Geometry check sheet. Reference: the model listing, model coordinates, mm. Coordinates: 2 decimals unless noted, no trailing zeros. Write each loop counter-clockwise with the first axis right and the second up, starting at its lowest first coordinate (ties: lowest second). Pieces come first, ordered by that corner, then holes.
from build123d import *

# Parameters (mm, degrees)
SKETCH1_W           = 15
SKETCH1_H           = 220
SKETCH1_W_2         = 519.948861259
SKETCH1_H_2         = 15
BOSS_EXTRUDE1_DEPTH = 20
BOSS_EXTRUDE3_DEPTH = 110
SKETCH3_R           = 7.5
CUT_EXTRUDE1_DEPTH  = 655.346046928
BOSS_EXTRUDE5_DEPTH = 10


with BuildPart() as part:
    # Sketch1 → Boss-Extrude1 (new body)
    with BuildSketch(Plane(origin=(0, 0, 0), x_dir=(1, 0, 0), z_dir=(0, 1, 0))):
        with Locations((72.505405333, -7.5)):
            Rectangle(SKETCH1_W, SKETCH1_H)
        with Locations((607.454266592, 0)):
            Rectangle(SKETCH1_W, SKETCH1_H)
        with Locations((339.979835963, 72.5)):
            Rectangle(SKETCH1_W_2, SKETCH1_H_2)
        with Locations((339.979835963, -87.5)):
            Rectangle(SKETCH1_W_2, SKETCH1_H_2)
    extrude(amount=-BOSS_EXTRUDE1_DEPTH)

    # Sketch2 → Boss-Extrude3 (add, symmetric)
    with BuildSketch(Plane.XY):
        with BuildLine():
            Line((145.005405333, 0), (185.005405333, 0))
            Line((185.005405333, 0), (185.005405333, -20))
            ThreePointArc((185.005405333, -20), (165.005392368, -39.99997407), (145.005405333, -19.99997407))
            Line((145.005405333, -19.99997407), (145.005405333, 0))
        make_face()
        with BuildLine():
            Line((494.954266592, 0), (534.954266592, 0))
            Line((534.954266592, 0), (534.954266592, -20))
            ThreePointArc((534.954266592, -20), (514.954261153, -39.999989122), (494.954266592, -19.999989122))
            Line((494.954266592, -19.999989122), (494.954266592, 0))
        make_face()
    extrude(amount=BOSS_EXTRUDE3_DEPTH, both=True)

    # Sketch3 → Cut-Extrude1 (cut, through all)
    with BuildSketch(Plane.XY.offset(110)):
        with Locations((165.005405333, -19.99997407)):
            Circle(SKETCH3_R)
        with Locations((514.954266592, -19.999989122)):
            Circle(SKETCH3_R)
    extrude(amount=-CUT_EXTRUDE1_DEPTH, mode=Mode.SUBTRACT)

    # Sketch4 → Boss-Extrude5 (add)
    with BuildSketch(Plane(origin=(0, 0, 0), x_dir=(1, 0, 0), z_dir=(0, 1, 0))):
        with BuildLine():
            Line((158.022043154, -30), (158.022043154, 30))
            ThreePointArc((158.022043154, 30), (163.022043154, 35), (168.022043154, 30))
            Line((168.022043154, 30), (168.022043154, -30))
            ThreePointArc((168.022043154, -30), (163.022043154, -35), (158.022043154, -30))
        make_face()
        with BuildLine():
            Line((508.880344162, -30), (508.880344162, 30))
            ThreePointArc((508.880344162, 30), (513.880344162, 35), (518.880344162, 30))
            Line((518.880344162, 30), (518.880344162, -30))
            ThreePointArc((518.880344162, -30), (513.880344162, -35), (508.880344162, -30))
        make_face()
    extrude(amount=BOSS_EXTRUDE5_DEPTH)


solid = part.part
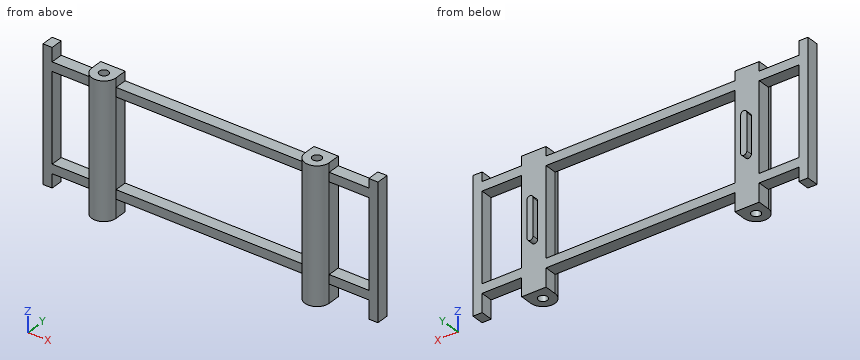
1. Gauge pin test, flat ends, axial feed: pin 1 Ø16 at (x, y) = (363.5, -9.5) entering from -Z; pin 2 Ø16 at (x, y) = (412.5, -13) entering from +Z; pin 3 Ø2 at (x, z) = (183, -85) entering from -Y. Record the tip position at first contact, or that the pin passes through.
Computed values:
pin 1: stops at z = -80
pin 2: stops at z = 95
pin 3: stops at y = -30.54
2. Sectioned sample at C-C, the plane z = -70. Record the boundary of the cut face in (x, y).
Computed values:
outline: (65.01, -20) - (145.01, -20) arc R20 ccw to (185.01, -20) - (494.95, -20) arc R20 ccw to (534.95, -20) - (614.95, -20) - (614.95, 0) - (65.01, 0) - close; hole circle Ø15 at (165.01, -20); hole circle Ø15 at (514.95, -20)
3. Sectioned sample at A-A, the plane z = -23. Record the boundary of the cut face in (x, y), and give its area (3 significant figures).
Computed values:
outline: (65.01, -20) - (80.01, -20) - (80.01, 0) - (65.01, 0) - close; (145.01, -20) arc R20 ccw to (185.01, -20) - (185.01, 0) - (168.02, 0) - (168.02, 10) - (158.02, 10) - (158.02, 0) - (145.01, 0) - close; (494.95, -20) arc R20 ccw to (534.95, -20) - (534.95, 0) - (518.88, 0) - (518.88, 10) - (508.88, 10) - (508.88, 0) - (494.95, 0) - close; (599.95, -20) - (614.95, -20) - (614.95, 0) - (599.95, 0) - close; hole circle Ø15 at (165.01, -20); hole circle Ø15 at (514.95, -20)
area: 3,300 mm2
4. Sectioned sample at B-B, the plane x = 479. Record the boundary of the cut face in (y, z), and give its area (3 significant figures).
Computed values:
outline: (-20, -80) - (0, -80) - (0, -65) - (-20, -65) - close; (-20, 80) - (0, 80) - (0, 95) - (-20, 95) - close
area: 600 mm2
5. Thickness scan on line 1 along X through (y, z) = (-6, 104); line 2 along X through (y, z) = (-21, -92); line 3 along Z through (x, y) = (586.5, -7.5). Record the ranges inside material, lowest first.
Computed values:
line 1: x = 65.01 to 80.01, 145.01 to 185.01, 494.95 to 534.95, 599.95 to 614.95
line 2: x = 145.03 to 157.57, 172.44 to 184.98, 494.98 to 507.52, 522.39 to 534.93
line 3: z = -80 to -65, 80 to 95
